Here's how the part is built. I have some questions about the finished solid (model axes, mm). Coordinates: 2 decimals unless noted, no trailing zeros. Loops run counter-clockwise (first coordinate to the right, second up) from the corner with the lowest first, then second, coordinate; pieces in that order, holes last. Notation, with made-up numbers: M -22.75,66.25 L 28.25,66.25 A7 ccw 28.25,72.25 Z; hole C -21.5,28 d8. An arc over 180 degrees is marked long. Use CSV: the item, a comma, the result in double quotes. Start each with the question number.
Q1. If we section it at D-D (y = -7): Please give me the cut outline in (x, z), and give its area (3 significant figures).
Q2. For pin 1 Ø2 at (x, z) = (-18.5, -0.5) entering from -Y; pin 2 Ø10 at (x, y) = (-24.5, 22.5) entering from -Z, each with a flat end and sliding along its axis, tell me the tip position at first contact or that it passes through.
Q3. If we section it at B-B (x = -8.5): Please give me the cut outline in (y, z).
Q4. If we section it at A-A (y = -18): Please give me the cut outline in (x, z).
Q5. If we mould it in two halves opening along Y, with no side actions, what happens to faces 1 (the cylindrical face through (-22.68, 28.52, 1.55)), 2 (the flat face through (-5, -21.753, 0)), 3 (the flat face through (-35.56, 26, 0)), 4 (the cylindrical face through (-5.01, -19.21, 0.11))? For each: +Y half, -Y half, draft (parallel to the pull), parting line (faces both ways), or undercut.
Q6. Please list where these lines run through material, in increasing order: probe 1 along X at (y, z) = (-14, -3.5); probe 2 along Y at (x, z) = (-2.5, -0.75); probe 3 along Y at (x, z) = (-15, 1). Write a range as [from, to].
Q7. If we section it at C-C (x = -24): Please give me the cut outline in (y, z).
from build123d import *

# Parameters (mm, degrees)
F1_DEPTH = 35.56
F0_R     = 2.54
F2_DEPTH = 10.16
F3_DEPTH = 10.16


with BuildPart() as f1:
    # F0 (on Right) → F1 (new body)
    with BuildSketch(Plane.YZ):
        with BuildLine():
            ThreePointArc((29.046643, 0), (26.506643, 2.54), (23.966643, 0))
            ThreePointArc((23.966643, 0), (26.506643, -2.54), (29.046643, 0))
        make_face()
    extrude(amount=-F1_DEPTH)

    # F0 (on Right) → F2 (join)
    with BuildSketch(Plane.YZ):
        Polygon((23.966643, 7.62), (-21.753357, 7.62), (-21.753357, -7.62), (23.966643, -7.62), (23.966643, 0), align=None)
        with Locations((-16.673357, 0)):
            Circle(F0_R, mode=Mode.SUBTRACT)
        with BuildLine():
            ThreePointArc((29.046643, 0), (26.506643, -2.54), (23.966643, 0))
            Line((23.966643, 0), (23.966643, -7.62))
            Line((23.966643, -7.62), (29.046643, -7.62))
            Line((29.046643, -7.62), (29.046643, 0))
        make_face()
    extrude(amount=-F2_DEPTH)

    # F0 (on Right) → F3 (join)
    with BuildSketch(Plane.YZ):
        with BuildLine():
            Line((29.046643, 7.62), (23.966643, 7.62))
            Line((23.966643, 7.62), (23.966643, 0))
            ThreePointArc((23.966643, 0), (26.506643, 2.54), (29.046643, 0))
            Line((29.046643, 0), (29.046643, 7.62))
        make_face()
    extrude(amount=-F3_DEPTH)


solid = f1.part
Results below:
1,outline,"M -10.16,-7.62 L 0,-7.62 L 0,7.62 L -10.16,7.62 Z"
1,area,"155 mm^2"
2,pin 1,"y = 23.97"
2,pin 2,"z = -2.54"
3,outline,"M -21.75,-7.62 L 29.05,-7.62 L 29.05,7.62 L -21.75,7.62 Z; hole C -16.67,0 d5.08"
4,outline,"M -10.16,-7.62 L 0,-7.62 L 0,-2.17 L -10.16,-2.17 Z; M -10.16,2.17 L 0,2.17 L 0,7.62 L -10.16,7.62 Z"
5,face 1,"parting line"
5,face 2,"-Y half"
5,face 3,"draft"
5,face 4,"undercut"
6,probe 1,"[-10.16, 0]"
6,probe 2,"[-21.75, -19.1], [-14.25, 29.05]"
6,probe 3,"[24.17, 28.84]"
7,outline,"C 26.51,0 d5.08"
